CAD build for the part. Positions are in the model's coordinates, mm. Round coordinates to 2 decimals unless told otherwise and drop trailing zeros. Order: outer loops, then holes, each group sorted by start corner. A loop starts at its lowest first (then second) coordinate and runs counter-clockwise, first axis right, second up. Notation, with made-up numbers: (18.25, -35.5) -> (25.25, -35.5) arc R21 ccw to (25.25, -8.5) -> close; hole circle Ø8 at (45.25, -23). An arc over 180 degrees is marked (long way). Return JSON: item names as keys, results as strings. Group by question number.
Q1. Cut at B-B (y = 5). Write the cut outline in (x, z).
Q2. Cut at D-D (y = 15). Write the cut outline in (x, z).
Q3. Mould opens along Z. For faces 1 (the flat face through (4, 9, -3)), 2 (the flat face through (1, 9, 23.65)), 3 (the cylindrical face through (0.704, 6.352, 3.176)) say: +Z half, -Z half, draft (parallel to the pull), parting line (faces both ways), or undercut.
Q4. Probe line 1 along Y through (x, z) = (-1.25, -27); line 2 along Y through (x, z) = (0.5, 4.65); line 3 along Z through (x, y) = (-0.5, 15). List the from-to ranges inside material, lowest first.
Q5. Cut at C-C (x = 3.5). Write the cut outline in (y, z), then the cut area to 3 significant figures.
Q6. Cut at A-A (z = 16.65). Write the cut outline in (x, y).
from build123d import *

# Parameters (mm, degrees)
BOSS_EXTRU_1_DEPTH      = 20
ESQUISSE3_W             = 4
ESQUISSE3_H             = 18
BOSS_EXTRU_2_DEPTH      = 20
ESQUISSE4_W             = 4
ESQUISSE4_H             = 18
BOSS_EXTRU_3_DEPTH      = 20
ESQUISSE5_W             = 17.65
ESQUISSE5_H             = 18
ESQUISSE5_W_2           = 16.35
ESQUISSE5_R             = 2
ENL_V_MAT_EXTRU_1_DEPTH = 20
ESQUISSE6_W             = 4
ESQUISSE6_H             = 26
BOSS_EXTRU_4_DEPTH      = 4
ESQUISSE7_R             = 2
ENL_V_MAT_EXTRU_2_DEPTH = 4
ESQUISSE8_R             = 2
ENL_V_MAT_EXTRU_3_DEPTH = 4
ESQUISSE9_W             = 4
ESQUISSE9_H             = 26
BOSS_EXTRU_5_DEPTH      = 8
ENL_V_MAT_EXTRU_5_DEPTH = 8
ESQUISSE13_W            = 20.25
ESQUISSE13_H            = 28
ENL_V_MAT_EXTRU_7_DEPTH = 46.255524525
ESQUISSE14_W            = 29
ESQUISSE14_H            = 22
ESQUISSE14_R            = 1.537122226
ESQUISSE14_R_2          = 1.624788677
BOSS_EXTRU_6_DEPTH      = 6.5
BOSS_EXTRU_7_START      = 2.5
ESQUISSE15_W            = 26
ESQUISSE15_H            = 22
ESQUISSE15_R            = 2
BOSS_EXTRU_7_DEPTH      = 2.5


with BuildPart() as part:
    # Esquisse1 → Boss.-Extru.1 (new body)
    with BuildSketch(Plane.XY):
        Polygon((0, 16), (0, 0), (24.25, 0), (24.25, 2), (4, 2), (4, 16), align=None)
        Polygon((24.25, 0), (0, 0), (0, -2), (20.25, -2), (20.25, -24), (24.25, -24), align=None)
    extrude(amount=BOSS_EXTRU_1_DEPTH)

    # Esquisse3 → Boss.-Extru.2 (add)
    with BuildSketch(Plane(origin=(0, 0, 0), x_dir=(-1, 0, 0), z_dir=(0, 0, -1))):
        with Locations((-2, 7)):
            Rectangle(ESQUISSE3_W, ESQUISSE3_H)
    extrude(amount=BOSS_EXTRU_2_DEPTH)

    # Esquisse4 → Boss.-Extru.3 (add)
    with BuildSketch(Plane.XY.offset(20)):
        with Locations((2, 7)):
            Rectangle(ESQUISSE4_W, ESQUISSE4_H)
    extrude(amount=BOSS_EXTRU_3_DEPTH)

    # Esquisse5 → Enlèv. mat.-Extru.1 (cut)
    with BuildSketch(Plane.ZY):
        with Locations((-11.175, 7)):
            Rectangle(ESQUISSE5_W, ESQUISSE5_H)
        with Locations((31.825, 7)):
            Rectangle(ESQUISSE5_W_2, ESQUISSE5_H)
        with Locations((16.65, 15)):
            Circle(ESQUISSE5_R)
        with Locations((4.65, 5)):
            Circle(ESQUISSE5_R)
    extrude(amount=-ENL_V_MAT_EXTRU_1_DEPTH, mode=Mode.SUBTRACT)

    # Esquisse6 → Boss.-Extru.4 (add)
    with BuildSketch(Plane(origin=(0, 16, 0), x_dir=(1, 0, 0), z_dir=(0, 1, 0))):
        with Locations((2, -10.65)):
            Rectangle(ESQUISSE6_W, ESQUISSE6_H)
    extrude(amount=BOSS_EXTRU_4_DEPTH)

    # Esquisse7 → Enlèv. mat.-Extru.2 (cut)
    with BuildSketch(Plane.ZY):
        with Locations((16.65, 15)):
            Circle(ESQUISSE7_R)
    extrude(amount=-ENL_V_MAT_EXTRU_2_DEPTH, mode=Mode.SUBTRACT)

    # Esquisse8 → Enlèv. mat.-Extru.3 (cut)
    with BuildSketch(Plane.ZY.offset(-20.25)):
        with Locations((20, -7)):
            Circle(ESQUISSE8_R)
        with Locations((20, -20)):
            Circle(ESQUISSE8_R)
    extrude(amount=-ENL_V_MAT_EXTRU_3_DEPTH, mode=Mode.SUBTRACT)

    # Esquisse9 → Boss.-Extru.5 (add)
    with BuildSketch(Plane.XY.offset(20)):
        with Locations((22.25, -11)):
            Rectangle(ESQUISSE9_W, ESQUISSE9_H)
    extrude(amount=BOSS_EXTRU_5_DEPTH)

    # Esquisse11 → Enlèv. mat.-Extru.5 (cut)
    with BuildSketch(Plane.ZY.offset(-20.25)):
        with BuildLine():
            ThreePointArc((20, -9), (21.414213562, -8.414213562), (22, -7))
            ThreePointArc((22, -7), (21.414213562, -5.585786438), (20, -5))
            Line((20, -5), (20, -9))
        make_face()
        with BuildLine():
            Line((20, -9), (20, -5))
            ThreePointArc((20, -5), (18, -7), (20, -9))
        make_face()
        with BuildLine():
            ThreePointArc((20, -22), (21.414213562, -21.414213562), (22, -20))
            ThreePointArc((22, -20), (21.414213562, -18.585786438), (20, -18))
            Line((20, -18), (20, -22))
        make_face()
        with BuildLine():
            Line((20, -22), (20, -18))
            ThreePointArc((20, -18), (18, -20), (20, -22))
        make_face()
        Polygon((14, -24), (0, -2), (0, -24), align=None)
    extrude(amount=-ENL_V_MAT_EXTRU_5_DEPTH, mode=Mode.SUBTRACT)

    # Esquisse13 → Enlèv. mat.-Extru.7 (cut, through all)
    with BuildSketch(Plane(origin=(0, 2, 0), x_dir=(1, 0, 0), z_dir=(0, 1, 0))):
        with Locations((14.125, -14)):
            Rectangle(ESQUISSE13_W, ESQUISSE13_H)
    extrude(amount=-ENL_V_MAT_EXTRU_7_DEPTH, mode=Mode.SUBTRACT)

    # Esquisse14 → Boss.-Extru.6 (add)
    with BuildSketch(Plane(origin=(4, 0, 0), x_dir=(0, 0, -1), z_dir=(1, 0, 0))):
        with Locations((16.85, 9)):
            Rectangle(ESQUISSE14_W, ESQUISSE14_H)
        with Locations(Location((27.18, 16, 0), (0, 0, 90))):
            Circle(ESQUISSE14_R, mode=Mode.SUBTRACT)
        with Locations(Location((27.18, 2, 0), (0, 0, 90))):
            Circle(ESQUISSE14_R_2, mode=Mode.SUBTRACT)
    extrude(amount=-BOSS_EXTRU_6_DEPTH)

    # Esquisse15 → Boss.-Extru.7 (add)
    with BuildSketch(Plane.ZY.offset(BOSS_EXTRU_7_START)):
        with Locations((10.65, 9)):
            Rectangle(ESQUISSE15_W, ESQUISSE15_H)
        with Locations((4.65, 5)):
            Circle(ESQUISSE15_R, mode=Mode.SUBTRACT)
        with Locations((16.65, 15)):
            Circle(ESQUISSE15_R, mode=Mode.SUBTRACT)
    extrude(amount=-BOSS_EXTRU_7_DEPTH)


solid = part.part
Solution:
{
 "1": {"outline": "(-2.5, -31.35) -> (4, -31.35) -> (4, 2.65) -> (-2.5, 2.65) -> close; (-2.5, 6.65) -> (4, 6.65) -> (4, 23.65) -> (-2.5, 23.65) -> close"},
 "2": {"outline": "(-2.5, -31.35) -> (4, -31.35) -> (4, -28.35) -> (-2.5, -28.35) -> close; (-2.5, -26.01) -> (4, -26.01) -> (4, 14.65) -> (-2.5, 14.65) -> close; (-2.5, 18.65) -> (4, 18.65) -> (4, 23.65) -> (-2.5, 23.65) -> close"},
 "3": {"face 1": "draft", "face 2": "+Z half", "face 3": "undercut"},
 "4": {"line 1": "y = -2 to 0.39, 3.61 to 14.47, 17.53 to 20", "line 2": "y = -2 to 3, 7 to 20", "line 3": "z = -31.35 to -28.35, -26.01 to 14.65, 18.65 to 23.65"},
 "5": {"outline": "(-2, -31.35) -> (20, -31.35) -> (20, 23.65) -> (-2, 23.65) -> close; hole circle Ø3.25 at (2, -27.18); hole circle Ø4 at (5, 4.65); hole circle Ø4 at (15, 16.65); hole circle Ø3.07 at (16, -27.18)", "area": "1,170 mm²"},
 "6": {"outline": "(-2.5, -2) -> (4, -2) -> (4, 13) -> (-2.5, 13) -> close; (-2.5, 17) -> (4, 17) -> (4, 20) -> (-2.5, 20) -> close"}
}
